The drawing under review shows one solid part. Ordinate dimensions are in mm from its lowest x, y, z. Round coordinates to 2 decimals unless told otherwise and drop trailing zeros. Order: outer loops, then holes, each group sorted by start corner. A loop starts at its lowest first (then second) coordinate and runs counter-clockwise, first axis right, second up.
1) Consider section A-A (z = 76.2). Give the boundary of the cut face in (x, y) (3 decimals), then the cut area to 3 significant figures.
2) Consider section C-C (z = 111). Give the boundary of the cut face in (x, y).
3) Consider section D-D (x = 82). Give the boundary of the cut face in (y, z).
4) To check wall thickness, follow L1, parallel to X at y = 2.5, z = 76.2 (3 decimals); L2, parallel to X at y = 1.25, z = 6 (3 decimals); L3, parallel to Z at x = 51.5, y = 1.75. State the ranges of each line that lie inside material, in increasing order.
5) Consider section B-B (y = 3.75). Give the boundary of the cut face in (x, z) (3 decimals), then the cut area to 3 significant figures.
6) Clearance check with flat-ended pins moving along their axes: P1, Ø1.9, axis at y = 3, z = 18, coming from the -X side (3 decimals); P2, Ø2, axis at x = 32, y = 1.5, coming from the -Z side; P3, Ø1.5, axis at y = 2.5, z = 86.5, coming from the -X side; P4, Ø1, axis at x = 62, y = 3, coming from the +Z side. State where each tip first meets the part, or that it passes through.
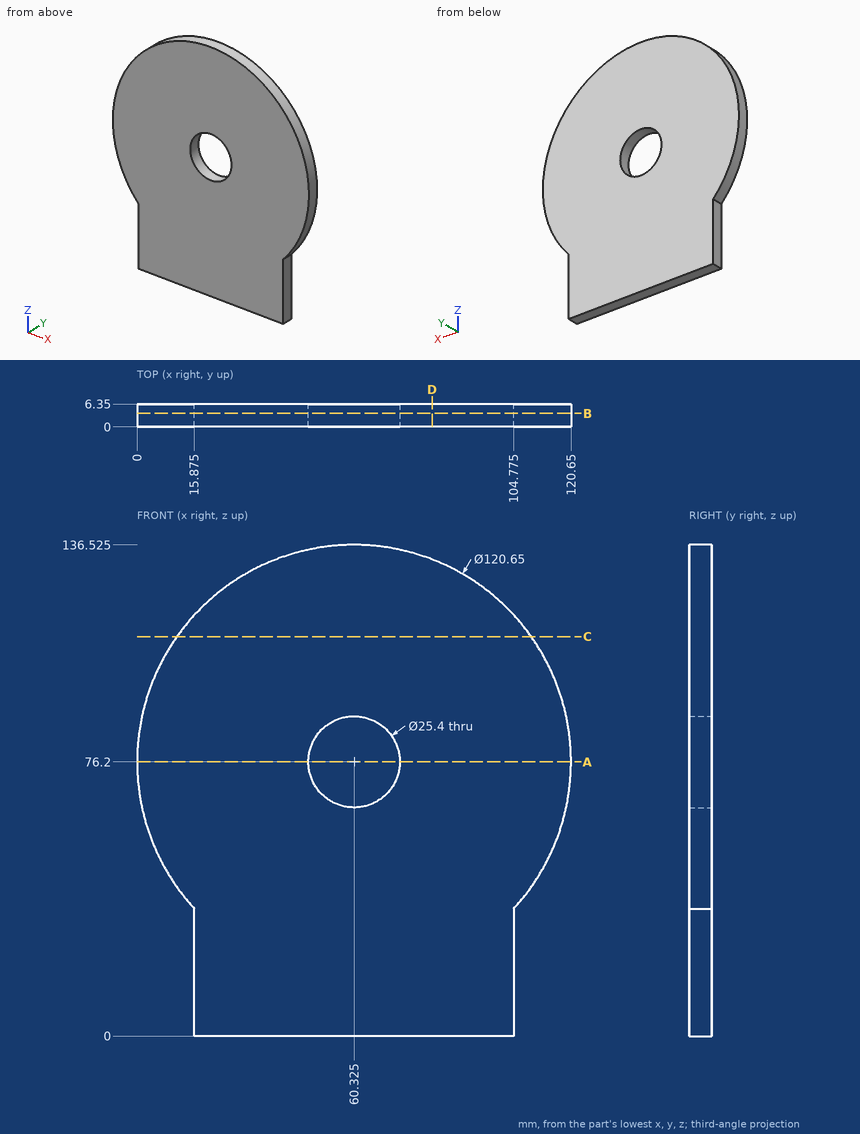
Answer below:
1. outline: (0, 0) - (47.625, 0) - (47.625, 6.35) - (0, 6.35) - close; (73.025, 0) - (120.65, 0) - (120.65, 6.35) - (73.025, 6.35) - close
1. area: 605 mm2
2. outline: (11.05, 0) - (109.6, 0) - (109.6, 6.35) - (11.05, 6.35) - close
3. outline: (0, 0) - (6.35, 0) - (6.35, 132.5) - (0, 132.5) - close
4. L1: x = 0 to 47.625, 73.025 to 120.65
4. L2: x = 15.875 to 104.775
4. L3: z = 0 to 67.07, 85.33 to 135.88
5. outline: (15.875, 0) - (104.775, 0) - (104.775, 35.416) arc R60.325 ccw (long way) to (15.875, 35.416) - close; hole circle Ø25.4 at (60.325, 76.2)
5. area: 12,900 mm2
6. P1: stops at x = 15.875
6. P2: stops at z = 0
6. P3: stops at x = 0.76
6. P4: stops at z = 136.51
